Can you work these out from the model? Positions are in its coordinate system, mm. A direction names the side the tool comes from. Give positions to 0.01 mm unless a question says otherwise; leave off trailing zeros. Order: outer loops, then holes, each group sorted by start corner. A loop starts at its lowest first (then second) coordinate and runs counter-clockwise, first axis right, second up. Notation, with made-up numbers: M 55,89 L 113,89 A10 ccw 113,93 Z; hole C 62.5,28 d4. An arc over 180 degrees is marked long. One line per question, with ' | ' between items. Start each with the question number.
1) If we section it at A-A, the plane y = 1.75: Please give me the cut outline in (x, z), plus the area to 3 significant figures.
2) Thinking about a two-plate mould opening in X: for faces 3 (the flat face through (-2.54, 4, 1)), 4 (the flat face through (-1, 4, 0.27)), 5 (the flat face through (-1, 4, 2.54)), which applies, +X half, -X half, draft (parallel to the pull), parting line (faces both ways), or undercut?
3) Please list where these lines run through material, in increasing order: line 1 along Z through (x, y) = (-0.9, 7); line 2 along X through (y, z) = (4.75, 2); line 3 along Y through (x, z) = (-1.2, 0.3). Write a range as [from, to].
4) For faces 1 (the flat face through (-0.75, 4, 1)), 2 (the flat face through (-1, 4, 0)), which set-ups out of +Z, -Z, +X, -X, +Y, -Y let a thin tool reach every point of the face, with its end or its side?
```python
from build123d import *

# Parameters (mm, degrees)
BOSS_EXTRUDE1_DEPTH = 2.54
SKETCH2_W           = 1.04
SKETCH2_H           = 2
CUT_EXTRUDE1_DEPTH  = 7
SKETCH3_W           = 1.54
SKETCH3_H           = 1.54
CUT_EXTRUDE2_DEPTH  = 0.5
CUT_EXTRUDE2_TAPER  = 27


with BuildPart() as part:
    # Sketch1 → Boss-Extrude1 (new body)
    with BuildSketch(Plane.XY):
        Polygon((-1.79, 0), (-2.54, 0), (-2.54, 8.5), (0, 8.5), (0, 0), (-0.75, 0), (-0.75, 1), (-1.79, 1), align=None)
    extrude(amount=BOSS_EXTRUDE1_DEPTH)

    # Sketch2 → Cut-Extrude1 (cut)
    with BuildSketch(Plane.XZ.offset(-1)):
        with Locations((-1.27, 1.27)):
            Rectangle(SKETCH2_W, SKETCH2_H)
    extrude(amount=-CUT_EXTRUDE1_DEPTH, mode=Mode.SUBTRACT)

    # Sketch3 → Cut-Extrude2 (cut)
    with BuildSketch(Plane(origin=(0, 8.5, 0), x_dir=(1, 0, 0), z_dir=(0, 1, 0))):
        with Locations((-1.27, -1.27)):
            Rectangle(SKETCH3_W, SKETCH3_H)
    extrude(amount=-CUT_EXTRUDE2_DEPTH, taper=CUT_EXTRUDE2_TAPER, mode=Mode.SUBTRACT)


solid = part.part
```
Results found:
1) outline: M -2.54,0 L 0,0 L 0,2.54 L -2.54,2.54 Z; hole M -1.79,0.27 L -0.75,0.27 L -0.75,2.27 L -1.79,2.27 Z | area: 4.37 mm²
2) face 3: -X half | face 4: undercut | face 5: draft
3) line 1: z = [0, 0.27], [2.27, 2.54] | line 2: x = [-2.54, -1.79], [-0.75, 0] | line 3: y = [8, 8.5]
4) face 1: -Y | face 2: -Z, +X, -X, +Y, -Y
